CAD build for the part. Positions are in the model's coordinates, mm. A direction names the side the tool comes from. Coordinates: 2 decimals unless noted, no trailing zeros. Order: outer loops, then holes, each group sorted by start corner. A loop starts at its lowest first (then second) coordinate and runs counter-clockwise, first axis right, second up. Notation, with made-up numbers: (36.5, -14) - (72.5, -14) arc R14 ccw to (72.5, -5) - close; hole circle Ø7 at (-3, -25). An arc over 180 degrees is marked (long way). Write each question's results on one line, items separated by ' | '. Start each with the question number.
Q1. Wall check: probe 1 along Z at (x, y) = (364, -6.75); probe 2 along Z at (x, y) = (424, -5.25); probe 3 along X at (y, z) = (-5.25, 768). Give the ranges that are in metal, low to high.
Q2. Which spindle directions (+Z, -Z, +X, -X, +Y, -Y) get a long thin tool onto all of the face, cutting with end or side? Do faces 5 (the flat face through (38, -9, 158)), 6 (the flat face through (222, 0, 477)), 7 (the flat face through (431, -9, 88)). Say none if no direction does.
Q3. Band-saw the part on A-A, the plane x = 331.5. Write the cut outline in (y, z), then the cut area to 3 significant figures.
Q4. Band-saw the part on D-D, the plane z = 674.5. Write the cut outline in (x, y).
Q5. Band-saw the part on C-C, the plane y = -3. Count the separate pieces of the cut face and the enclosed holes in it, then the cut area to 3 significant figures.
Q6. Band-saw the part on B-B, the plane z = 161. Write the cut outline in (x, y).
Q7. Pin check, flat tips, straight feed: P1, Ø6.5, axis at y = -8.5, z = 912.5, coming from the +X side; P2, Ø4, axis at y = -8, z = 28.5, coming from the +X side; P3, Ø4, axis at y = -15.5, z = 630, coming from the +X side. Stop position of each tip, or through.
Q8. Pull direction Z, two halves, no side cores. Call faces 1 (the flat face through (231, -9, 940)), 2 (the flat face through (0, -9, 476)), 3 (the flat face through (224, -9, 0)), 4 (the flat face through (302, -9, 20)): released by +Z, released by -Z, zero draft, split by the parting line, or undercut.
```python
from build123d import *

# Parameters (mm, degrees)
F1_DEPTH = 18
F2_W     = 18
F2_H     = 80
F3_DEPTH = 25
F4_R     = 10
F5_R     = 5
F6_R     = 5
F7_R     = 5


# Not quite as in the source:
# - two fillets or chamfers of one size are made in one step


with BuildPart() as f1:
    # F0 (on Front) → F1 (new body)
    with BuildSketch(Plane.XZ):
        Polygon((0, 940), (0, 0), (450, 0), (450, 20), (150, 20), (150, 38), (412, 38), (412, 88), (450, 88), (450, 188), (412, 188), (412, 752), (450, 752), (450, 852), (412, 852), (412, 902), (150, 902), (150, 920), (450, 920), (450, 940), align=None)
    extrude(amount=F1_DEPTH)

    # F2 (on face) → F3 (cut)
    with BuildSketch(Plane.XZ.offset(18)):
        with Locations((29, 782)):
            Rectangle(F2_W, F2_H)
        with Locations((29, 158)):
            Rectangle(F2_W, F2_H)
    extrude(amount=-F3_DEPTH, mode=Mode.SUBTRACT)

    # F4
    f4_edges = [f1.edges().sort_by_distance(p)[0] for p in [
        (0, -9, 0),
        (0, -9, 940),
    ]]
    fillet(f4_edges, radius=F4_R)

    # F5
    f5_edges = [f1.edges().sort_by_distance(p)[0] for p in [
        (20, -9, 822),
        (38, -9, 822),
        (20, -9, 742),
        (38, -9, 742),
    ]]
    fillet(f5_edges, radius=F5_R)

    # F6
    f6_edges = [f1.edges().sort_by_distance(p)[0] for p in [
        (38, -9, 198),
        (20, -9, 198),
        (20, -9, 118),
        (38, -9, 118),
    ]]
    fillet(f6_edges, radius=F6_R)

    # F7
    f7_edges = [f1.edges().sort_by_distance(p)[0] for p in [
        (450, -9, 0),
        (450, -9, 20),
        (150, -9, 38),
        (150, -9, 20),
        (450, -9, 940),
        (450, -9, 920),
        (150, -9, 920),
        (150, -9, 902),
        (412, -9, 902),
        (412, -9, 38),
        (412, -9, 852),
        (412, -9, 88),
        (450, -9, 852),
        (450, -9, 88),
        (450, -9, 752),
        (450, -9, 188),
        (412, -9, 752),
        (412, -9, 188),
    ]]
    fillet(f7_edges, radius=F7_R)


solid = f1.part
```
Results below:
1) probe 1: z = 0 to 20, 38 to 902, 920 to 940 | probe 2: z = 0 to 20, 88 to 188, 752 to 852, 920 to 940 | probe 3: x = 0 to 20, 38 to 450
2) face 5: +Y, -Y | face 6: +Z, -Z, +X, -X, +Y | face 7: +X, +Y, -Y
3) outline: (-18, 0) - (0, 0) - (0, 20) - (-18, 20) - close; (-18, 38) - (0, 38) - (0, 902) - (-18, 902) - close; (-18, 920) - (0, 920) - (0, 940) - (-18, 940) - close | area: 16,300 mm²
4) outline: (0, -18) - (412, -18) - (412, 0) - (0, 0) - close
5) separate pieces: 1 | enclosed holes: 2 | area: 384,000 mm²
6) outline: (0, -18) - (20, -18) - (20, 0) - (0, 0) - close; (38, -18) - (450, -18) - (450, 0) - (38, 0) - close
7) P1: stops at x = 150.06 | P2: stops at x = 150 | P3: stops at x = 412
8) face 1: released by +Z | face 2: zero draft | face 3: released by -Z | face 4: undercut
